Could you check a few things on this model? Use its own coordinates, in mm. Face numbers are marked on the shaded views. A direction names the side the tool comes from. Round coordinates to 2 decimals unless told otherwise and drop trailing zeros. Loops run counter-clockwise (first coordinate to the right, second up) from the corner with the lowest first, then second, coordinate; pieces in that order, holes last. Notation, with made-up numbers: (67.5, 52.25) -> (85.5, 52.25) arc R16 ccw to (85.5, 71.25) -> close; hole circle Ø3 at (-6.5, 51.5). An arc over 180 degrees is marked (long way). One line per item, written item: value.
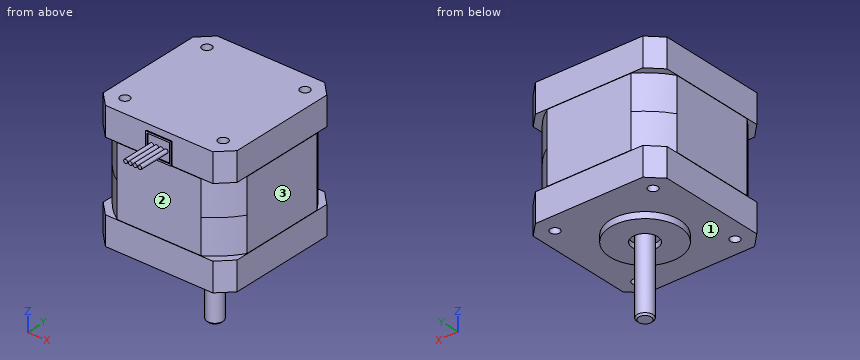
```python
from build123d import *

# Parameters (mm, degrees)
ESQUISSE1_R             = 1.5
EXTRUSION1_DEPTH        = 40
ESQUISSE10_W            = 8
ESQUISSE10_H            = 7
ESQUISSE10_W_2          = 7
ESQUISSE10_H_2          = 6
BOSS_EXTRU_2_DEPTH      = 0.3
ESQUISSE2_R             = 11
EXTRUSION2_DEPTH        = 2
ESQUISSE3_R             = 2.5
EXTRUSION3_DEPTH        = 22
ENL_V_START             = -1.6
ESQUISSE4_R             = 4
ESQUISSE4_R_2           = 2.5
ENL_V_MAT_EXTRU_1_DEPTH = 1.6
CHANFREIN1_SIZE         = 0.5
ESQUISSE6_R             = 34.95
ESQUISSE6_R_2           = 24.95
ENL_V_MAT_EXTRU_3_DEPTH = 11
ESQUISSE7_R             = 25.05
ESQUISSE7_R_2           = 19.05
ENL_V_MAT_EXTRU_4_DEPTH = 0.1
SYM_TRIE1_START         = 20
SYM_TRIE1_DEPTH         = 11
SYM_TRIE1_START_2       = 30.9
SYM_TRIE1_2_OUTLINE_R   = 1.5
SYM_TRIE1_2_OUTLINE_R_2 = 19.05
SYM_TRIE1_2_DEPTH       = 0.1
ESQUISSE10_3_R          = 0.6
BOSS_EXTRU_3_DEPTH      = 10


# Read off the part's stored shape, not the designer's step: Symétrie1
with BuildPart() as part:
    # Esquisse1 → Extrusion1 (new body)
    with BuildSketch(Plane.XY):
        Polygon((-16.963055506, 21.15), (16.963055506, 21.15), (21.15, 16.963055506), (21.15, -16.963055506), (16.963055506, -21.15), (-16.963055506, -21.15), (-21.15, -16.963055506), (-21.15, 16.963055506), align=None)
        with Locations((-15.5, 15.5)):
            Circle(ESQUISSE1_R, mode=Mode.SUBTRACT)
        with Locations((15.5, -15.5)):
            Circle(ESQUISSE1_R, mode=Mode.SUBTRACT)
        with Locations(Location((-15.5, -15.5, 0), (0, 0, 180))):
            Circle(ESQUISSE1_R, mode=Mode.SUBTRACT)
        with Locations(Location((15.5, 15.5, 0), (0, 0, 180))):
            Circle(ESQUISSE1_R, mode=Mode.SUBTRACT)
    extrude(amount=EXTRUSION1_DEPTH)

    # Esquisse10 → Boss.-Extru.2 (add)
    with BuildSketch(Plane.XZ.offset(21.15)):
        with Locations((0, 34.5)):
            Rectangle(ESQUISSE10_W, ESQUISSE10_H)
        with Locations((0, 34.5)):
            Rectangle(ESQUISSE10_W_2, ESQUISSE10_H_2, mode=Mode.SUBTRACT)
    extrude(amount=BOSS_EXTRU_2_DEPTH)

    # Esquisse2 → Extrusion2 (add)
    with BuildSketch(Plane(origin=(0, 0, 0), x_dir=(-1, 0, 0), z_dir=(0, 0, -1))):
        with Locations(Location((0, 0, 0), (0, 0, 180))):
            Circle(ESQUISSE2_R)
    extrude(amount=EXTRUSION2_DEPTH)

    # Esquisse3 → Extrusion3 (add)
    with BuildSketch(Plane(origin=(0, 0, -2), x_dir=(-1, 0, 0), z_dir=(0, 0, -1))):
        Circle(ESQUISSE3_R)
    extrude(amount=EXTRUSION3_DEPTH)

    # Esquisse4 → Enlèv. mat.-Extru.1 (cut)
    with BuildSketch(Plane(origin=(0, 0, -2), x_dir=(-1, 0, 0), z_dir=(0, 0, -1)).offset(ENL_V_START)):
        Circle(ESQUISSE4_R)
        Circle(ESQUISSE4_R_2, mode=Mode.SUBTRACT)
    extrude(amount=ENL_V_MAT_EXTRU_1_DEPTH, mode=Mode.SUBTRACT)

    # Chanfrein1
    chanfrein1_edges = [part.edges().sort_by_distance(p)[0] for p in [
        (2.5, 0, -24),
    ]]
    chamfer(chanfrein1_edges, length=CHANFREIN1_SIZE)

    # Esquisse6 → Enlèv. mat.-Extru.3 (cut)
    with BuildSketch(Plane(origin=(0, 0, 9), x_dir=(-1, 0, 0), z_dir=(0, 0, -1))):
        Circle(ESQUISSE6_R)
        Circle(ESQUISSE6_R_2, mode=Mode.SUBTRACT)
    extrude(amount=-ENL_V_MAT_EXTRU_3_DEPTH, mode=Mode.SUBTRACT)

    # Esquisse7 → Enlèv. mat.-Extru.4 (cut)
    with BuildSketch(Plane(origin=(0, 0, 9), x_dir=(-1, 0, 0), z_dir=(0, 0, -1))):
        Circle(ESQUISSE7_R)
        Circle(ESQUISSE7_R_2, mode=Mode.SUBTRACT)
    extrude(amount=-ENL_V_MAT_EXTRU_4_DEPTH, mode=Mode.SUBTRACT)

    # Symétrie1 outline → Symétrie1 (cut)
    with BuildSketch(Plane.XY.offset(SYM_TRIE1_START)):
        with BuildLine():
            Line((21.15, -16.963055506), (21.15, -13.235558167))
            ThreePointArc((21.15, -13.235558167), (17.642314191, -17.642314191), (13.235558167, -21.15))
            Line((13.235558167, -21.15), (16.963055506, -21.15))
            Line((16.963055506, -21.15), (21.15, -16.963055506))
        make_face()
        with BuildLine():
            ThreePointArc((13.235558167, 21.15), (17.642314191, 17.642314191), (21.15, 13.235558167))
            Line((21.15, 13.235558167), (21.15, 16.963055506))
            Line((21.15, 16.963055506), (16.963055506, 21.15))
            Line((16.963055506, 21.15), (13.235558167, 21.15))
        make_face()
        with BuildLine():
            Line((-16.963055506, -21.15), (-13.235558167, -21.15))
            ThreePointArc((-13.235558167, -21.15), (-17.642314191, -17.642314191), (-21.15, -13.235558167))
            Line((-21.15, -13.235558167), (-21.15, -16.963055506))
            Line((-21.15, -16.963055506), (-16.963055506, -21.15))
        make_face()
        with BuildLine():
            ThreePointArc((-21.15, 13.235558167), (-17.642314191, 17.642314191), (-13.235558167, 21.15))
            Line((-13.235558167, 21.15), (-16.963055506, 21.15))
            Line((-16.963055506, 21.15), (-21.15, 16.963055506))
            Line((-21.15, 16.963055506), (-21.15, 13.235558167))
        make_face()
    extrude(amount=SYM_TRIE1_DEPTH, mode=Mode.SUBTRACT)

    # Sym_trie1 2 outline → Sym_trie1 2 (cut)
    with BuildSketch(Plane.XY.offset(SYM_TRIE1_START_2)):
        with BuildLine():
            ThreePointArc((13.235558167, -21.15), (17.642314191, -17.642314191), (21.15, -13.235558167))
            Line((21.15, -13.235558167), (21.15, 13.235558167))
            ThreePointArc((21.15, 13.235558167), (17.642314191, 17.642314191), (13.235558167, 21.15))
            Line((13.235558167, 21.15), (-13.235558167, 21.15))
            ThreePointArc((-13.235558167, 21.15), (-17.642314191, 17.642314191), (-21.15, 13.235558167))
            Line((-21.15, 13.235558167), (-21.15, -13.235558167))
            ThreePointArc((-21.15, -13.235558167), (-17.642314191, -17.642314191), (-13.235558167, -21.15))
            Line((-13.235558167, -21.15), (13.235558167, -21.15))
        make_face()
        with Locations((-15.5, -15.5)):
            Circle(SYM_TRIE1_2_OUTLINE_R, mode=Mode.SUBTRACT)
        with Locations((15.5, -15.5)):
            Circle(SYM_TRIE1_2_OUTLINE_R, mode=Mode.SUBTRACT)
        with Locations((-15.5, 15.5)):
            Circle(SYM_TRIE1_2_OUTLINE_R, mode=Mode.SUBTRACT)
        Circle(SYM_TRIE1_2_OUTLINE_R_2, mode=Mode.SUBTRACT)
        with Locations((15.5, 15.5)):
            Circle(SYM_TRIE1_2_OUTLINE_R, mode=Mode.SUBTRACT)
    extrude(amount=SYM_TRIE1_2_DEPTH, mode=Mode.SUBTRACT)

    # Esquisse10<3> → Boss.-Extru.3 (add)
    with BuildSketch(Plane.XZ.offset(21.15)):
        with Locations(Location((2.25, 34.5, 0), (0, 0, 90))):
            Circle(ESQUISSE10_3_R)
        with Locations(Location((0.75, 34.5, 0), (0, 0, 90))):
            Circle(ESQUISSE10_3_R)
        with Locations(Location((-0.75, 34.5, 0), (0, 0, 90))):
            Circle(ESQUISSE10_3_R)
        with Locations(Location((-2.25, 34.5, 0), (0, 0, 90))):
            Circle(ESQUISSE10_3_R)
    extrude(amount=BOSS_EXTRU_3_DEPTH)


solid = part.part
```
Item 1: If we section it at D-D on x = -15.5: Count the separate pieces of the cut face and the enclosed holes in it, plus the area to 3 significant figures.
Output:
separate pieces: 7
enclosed holes: 0
area: 1,380 mm²
Item 2: If we section it at C-C on x = -5.5: List the corners of the cut face in (y, z) for me, plus the area to 3 significant figures.
Output:
outline: (-21.15, 0) -> (-9.53, 0) -> (-9.53, -2) -> (9.53, -2) -> (9.53, 0) -> (21.15, 0) -> (21.15, 9) -> (18.24, 9) -> (18.24, 9.1) -> (21.15, 9.1) -> (21.15, 30.9) -> (18.24, 30.9) -> (18.24, 31) -> (21.15, 31) -> (21.15, 40) -> (-21.15, 40) -> (-21.15, 31) -> (-18.24, 31) -> (-18.24, 30.9) -> (-21.15, 30.9) -> (-21.15, 9.1) -> (-18.24, 9.1) -> (-18.24, 9) -> (-21.15, 9) -> close
area: 1,730 mm²
Item 3: If we section it at A-A on z = 21: List the corners of the cut face in (x, y) for me, plus the area to 3 significant figures.
Output:
outline: (-21.15, -13.24) arc R24.95 ccw to (-13.24, -21.15) -> (13.24, -21.15) arc R24.95 ccw to (21.15, -13.24) -> (21.15, 13.24) arc R24.95 ccw to (13.24, 21.15) -> (-13.24, 21.15) arc R24.95 ccw to (-21.15, 13.24) -> close; hole circle Ø3 at (-15.5, -15.5); hole circle Ø3 at (-15.5, 15.5); hole circle Ø3 at (15.5, -15.5); hole circle Ø3 at (15.5, 15.5)
area: 1,650 mm²
Item 4: I need wall thicknesses on line 1 (X direction, y = 15.5, z = 6.5); line 2 (Y direction, x = -14.5, z = 26). Which ranges of each line are inside material? Lowest first, please. Write a range as from..to.
Output:
line 1: x = -21.15..-17, -14..14, 17..21.15
line 2: y = -20.3..-16.62, -14.38..14.38, 16.62..20.3
Item 5: For the marked faces 1, 2 and 3, which set-ups out of +Z, -Z, +X, -X, +Y, -Y let a thin tool reach every point of the face, with its end or its side?
Output:
face 1: -Z
face 2: -Z, +X, -X, -Y
face 3: +Z, -Z, +X, +Y, -Y
Item 6: Will these pins go through, and if not, where does the flat tip stop? pin 1 Ø4 at (x, y) = (15.5, 15.5) entering from -Z; pin 2 Ø5 at (y, z) = (-22, 13) entering from +X; pin 3 Ø4.5 at (x, z) = (2.5, 3) entering from -Y.
Output:
pin 1: stops at z = 0
pin 2: stops at x = 15.56
pin 3: stops at y = -21.15
